Study the drawing (mm; zero at the part's minimum x, y, z) and answer. Give positions to 0.01 mm unless a question says otherwise; leave off trailing zeros. Loops run counter-clockwise (first coordinate to the right, second up) from the corner with the lowest first, then second, coordinate; pieces in that order, holes last. Notation, with made-up numbers: (-14, -3.75) - (24, -3.75) arc R19 ccw to (24, 7.25) - close; hole circle Ø10 at (50.25, 61). An arc over 180 degrees is marked (long way). Use one line per item in the form item = value. Start each with the question number.
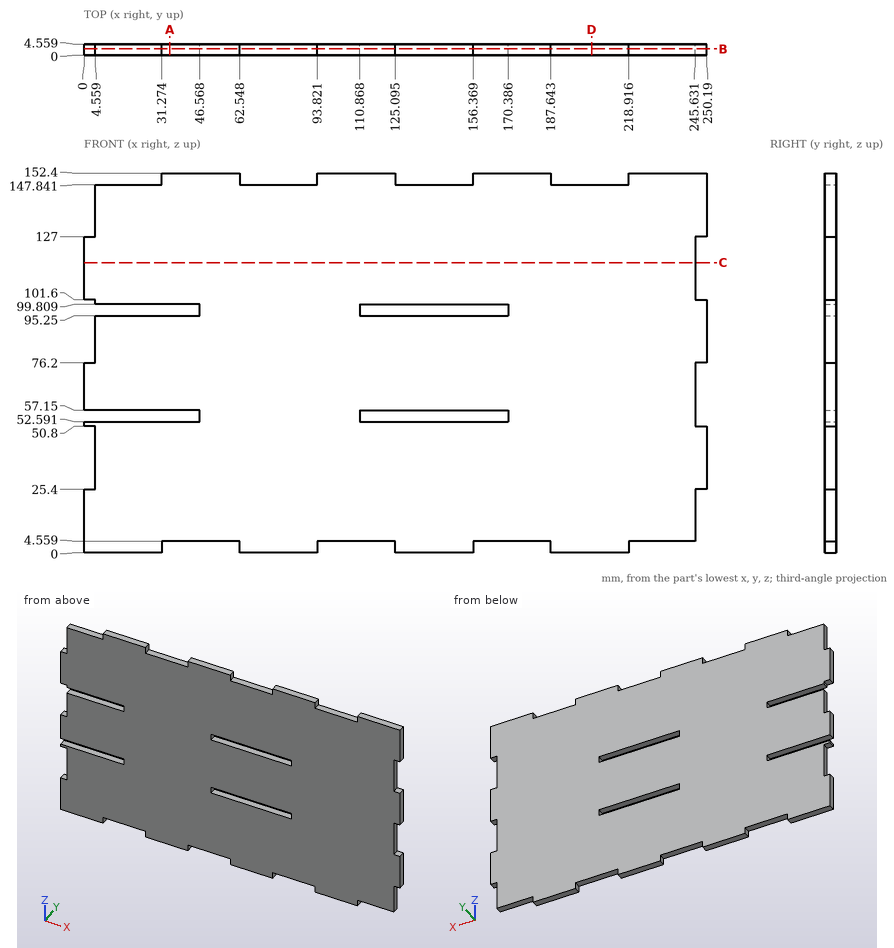
1) A cutting plane is placed at A-A (x = 34.5). Give the vertices of the cut face in (y, z).
2) A cutting plane is placed at C-C (z = 116.5). Give the vertices of the cut face in (x, y), plus the area to 3 significant figures.
3) A cutting plane is placed at D-D (x = 204). Give the vertices of the cut face in (y, z), plus the area to 3 significant figures.
4) A cutting plane is placed at B-B (y = 2.6). State how many separate pieces and enclosed holes the cut face has, plus the area to 3 significant figures.
5) Find the intervals of material crossed by probe 1 along Z at (x, y) = (149.5, 3); probe 2 along Z at (x, y) = (170, 1.7); probe 3 along X at (y, z) = (3.85, 96), in increasing order.
6) Flat-ended cylindrical pins translate along their axes: pin 1 Ø1.4 at (x, y) = (2, 1) entering from +Z; pin 2 Ø12 at (x, z) = (66.5, 113.5) entering from -Y; pin 3 Ø1.4 at (y, z) = (2, 2.5) entering from +X; pin 4 Ø2.5 at (y, z) = (2.5, 87.5) entering from -X. Find the tip coordinate at first contact, or state that the pin passes through.
Answer sheet:
q1.outline = (0, 4.56) - (4.56, 4.56) - (4.56, 52.59) - (0, 52.59) - close; (0, 57.15) - (4.56, 57.15) - (4.56, 95.25) - (0, 95.25) - close; (0, 99.81) - (4.56, 99.81) - (4.56, 152.4) - (0, 152.4) - close
q2.outline = (0, 0) - (245.63, 0) - (245.63, 4.56) - (0, 4.56) - close
q2.area = 1,120 mm²
q3.outline = (0, 0) - (4.56, 0) - (4.56, 147.84) - (0, 147.84) - close
q3.area = 674 mm²
q4.separate_pieces = 1
q4.enclosed_holes = 2
q4.area = 35,400 mm²
q5.probe_1 = 0 to 52.59, 57.15 to 95.25, 99.81 to 147.84
q5.probe_2 = 4.56 to 52.59, 57.15 to 95.25, 99.81 to 152.4
q5.probe_3 = 46.57 to 110.87, 170.39 to 250.19
q6.pin_1 = 127
q6.pin_2 = 0
q6.pin_3 = 218.92
q6.pin_4 = 4.56
